from build123d import *

# Parameters (mm, degrees)
BOSS_EXTRUDE1_DEPTH = 92
BOSS_EXTRUDE2_DEPTH = 11
BOSS_EXTRUDE3_DEPTH = 5
CUT_EXTRUDE1_REACH  = 91.375
SKETCH4_R           = 1.05
BOSS_EXTRUDE4_DEPTH = 11
CUT_EXTRUDE2_DEPTH  = 6.153427125
CUT_EXTRUDE3_REACH  = 96.249
SKETCH7_R           = 1.05
CHAMFER2_SIZE       = 2


with BuildPart() as part:
    # Sketch1 → Boss-Extrude1 (new body)
    with BuildSketch(Plane(origin=(0, 0, 0), x_dir=(1, 0, 0), z_dir=(0, 1, 0))):
        Polygon((0, 15.628427125), (-2.5, 15.628427125), (-13.153427125, 4.975), (-13.153427125, -5.025), (-2.5, -15.678427125), (0, -15.678427125), (0, -7.725), (-7.675, -7.725), (-7.675, 7.625), (0, 7.625), align=None)
    extrude(amount=BOSS_EXTRUDE1_DEPTH)

    # Sketch2 → Boss-Extrude2 (add)
    with BuildSketch(Plane.XZ):
        with BuildLine():
            Line((0, 7.725), (0, 5.075))
            ThreePointArc((0, 5.075), (-5.075, 0), (0, -5.075))
            Line((0, -5.075), (0, -7.625))
            Line((0, -7.625), (-7.675, -7.625))
            Line((-7.675, -7.625), (-7.675, 7.725))
            Line((-7.675, 7.725), (0, 7.725))
        make_face()
    extrude(amount=-BOSS_EXTRUDE2_DEPTH)

    # Sketch3 → Boss-Extrude3 (add)
    with BuildSketch(Plane(origin=(0, 92, 0), x_dir=(1, 0, 0), z_dir=(0, 1, 0))):
        Polygon((-2.5, 15.628427125), (-13.153427125, 15.628427125), (-13.153427125, 4.975), align=None)
        Polygon((-2.5, -15.678427125), (-13.153427125, -15.678427125), (-13.153427125, -5.025), align=None)
    extrude(amount=-BOSS_EXTRUDE3_DEPTH)

    # Sketch4 → Cut-Extrude1 (cut, up to next)
    with BuildSketch(Plane.XZ.offset(-87), mode=Mode.PRIVATE) as cut_extrude1_sk1:
        with Locations(Location((-10.153427125, 12.678427125, 0), (0, 0, 270))):
            Circle(SKETCH4_R)
    cut_extrude1_tool1 = extrude(cut_extrude1_sk1.sketch, amount=-CUT_EXTRUDE1_REACH, mode=Mode.PRIVATE) & part.part
    # Sketch4 → Cut-Extrude1 (cut, up to next)
    with BuildSketch(Plane.XZ.offset(-87), mode=Mode.PRIVATE) as cut_extrude1_sk2:
        with Locations(Location((-10.153427125, -12.628427125, 0), (0, 0, 270))):
            Circle(SKETCH4_R)
    cut_extrude1_tool2 = extrude(cut_extrude1_sk2.sketch, amount=-CUT_EXTRUDE1_REACH, mode=Mode.PRIVATE) & part.part
    add(cut_extrude1_tool1.solids().sort_by_distance((-10.153427, 87, 12.678427))[0], mode=Mode.SUBTRACT)
    add(cut_extrude1_tool2.solids().sort_by_distance((-10.153427, 87, -12.628427))[0], mode=Mode.SUBTRACT)

    # Sketch5 → Boss-Extrude4 (add)
    with BuildSketch(Plane.XZ):
        Polygon((-2.5, 15.678427125), (-13.153427125, 15.678427125), (-13.153427125, 5.025), align=None)
        Polygon((-13.153427125, -4.975), (-13.153427125, -15.628427125), (-2.5, -15.628427125), align=None)
    extrude(amount=-BOSS_EXTRUDE4_DEPTH)

    # Sketch6 → Cut-Extrude2 (cut)
    with BuildSketch(Plane.ZY.offset(13.153427125)):
        Polygon((11.564149128, 7.6), (9.139277997, 7.6), (7.926842432, 5.5), (9.139277997, 3.4), (11.564149128, 3.4), (12.776584693, 5.5), align=None)
        Polygon((-7.876842432, 5.5), (-9.089277997, 7.6), (-11.514149128, 7.6), (-12.726584693, 5.5), (-11.514149128, 3.4), (-9.089277997, 3.4), align=None)
    extrude(amount=-CUT_EXTRUDE2_DEPTH, mode=Mode.SUBTRACT)

    # Sketch7 → Cut-Extrude3 (cut, up to next)
    with BuildSketch(Plane.ZY.offset(13.153427125), mode=Mode.PRIVATE) as cut_extrude3_sk1:
        with Locations((-10.301713562, 5.5)):
            Circle(SKETCH7_R)
    cut_extrude3_tool1 = extrude(cut_extrude3_sk1.sketch, amount=-CUT_EXTRUDE3_REACH, mode=Mode.PRIVATE) & part.part
    # Sketch7 → Cut-Extrude3 (cut, up to next)
    with BuildSketch(Plane.ZY.offset(13.153427125), mode=Mode.PRIVATE) as cut_extrude3_sk2:
        with Locations((10.351713562, 5.5)):
            Circle(SKETCH7_R)
    cut_extrude3_tool2 = extrude(cut_extrude3_sk2.sketch, amount=-CUT_EXTRUDE3_REACH, mode=Mode.PRIVATE) & part.part
    add(cut_extrude3_tool1.solids().sort_by_distance((-13.153427, 5.5, -10.301714))[0], mode=Mode.SUBTRACT)
    add(cut_extrude3_tool2.solids().sort_by_distance((-13.153427, 5.5, 10.351714))[0], mode=Mode.SUBTRACT)

    # Chamfer2
    # the kernel refuses this chamfer: 2 mm, written as the material it takes off along each edge
    with BuildSketch(Plane(origin=(-7, 5.5, 10.351713562), x_dir=(0, 0, 1), z_dir=(0, -1, 0))) as chamfer2_piece_1_section:
        Polygon((1.05, -CHAMFER2_SIZE), (1.05 + CHAMFER2_SIZE, 0), (1.05, 0), align=None)
    chamfer2_piece_1 = revolve(axis=Axis((-7, 5.5, 10.351713562), (-1, 0, 0)), mode=Mode.PRIVATE)
    chamfer2_piece_1 = split(chamfer2_piece_1, bisect_by=Plane(origin=(-5.677336613, 7.282209745, 11.747625417), z_dir=(2.5539348178531628e-15, -0.5000000000000006, -0.8660254037844384)), keep=Keep.TOP, mode=Mode.PRIVATE)
    chamfer2_piece_1 = split(chamfer2_piece_1, bisect_by=Plane(origin=(-5.677336613, 3.717790255, 11.747625417), z_dir=(2.553934817853164e-15, 0.5000000000000003, -0.8660254037844387)), keep=Keep.TOP, mode=Mode.PRIVATE)
    chamfer2_piece_1 = split(chamfer2_piece_1, bisect_by=Plane(origin=(-5.677336613, 3.4, 8.660747588), z_dir=(0, 1, 0)), keep=Keep.TOP, mode=Mode.PRIVATE)
    chamfer2_piece_1 = split(chamfer2_piece_1, bisect_by=Plane(origin=(-5.677336613, 5.182209745, 8.110318721), z_dir=(-2.5539348178531624e-15, 0.5000000000000008, 0.8660254037844383)), keep=Keep.TOP, mode=Mode.PRIVATE)
    chamfer2_piece_1 = split(chamfer2_piece_1, bisect_by=Plane(origin=(-5.677336613, 5.817790255, 8.110318721), z_dir=(-2.5539348178531624e-15, -0.5000000000000007, 0.8660254037844384)), keep=Keep.TOP, mode=Mode.PRIVATE)
    chamfer2_piece_1 = split(chamfer2_piece_1, bisect_by=Plane(origin=(-5.677336613, 7.6, 8.660747588), z_dir=(0, -1, 0)), keep=Keep.TOP, mode=Mode.PRIVATE)
    add(chamfer2_piece_1, mode=Mode.SUBTRACT)
    with BuildSketch(Plane(origin=(-7, 5.5, -10.301713562), x_dir=(0, 0, 1), z_dir=(0, -1, 0))) as chamfer2_piece_2_section:
        Polygon((1.05, -CHAMFER2_SIZE), (1.05 + CHAMFER2_SIZE, 0), (1.05, 0), align=None)
    chamfer2_piece_2 = revolve(axis=Axis((-7, 5.5, -10.301713562), (-1, 0, 0)), mode=Mode.PRIVATE)
    chamfer2_piece_2 = split(chamfer2_piece_2, bisect_by=Plane(origin=(-5.677336613, 3.717790255, -8.905801708), z_dir=(2.5539348178531635e-15, 0.5000000000000004, -0.8660254037844385)), keep=Keep.TOP, mode=Mode.PRIVATE)
    chamfer2_piece_2 = split(chamfer2_piece_2, bisect_by=Plane(origin=(-5.677336613, 3.4, -11.992679537), z_dir=(0, 1, 0)), keep=Keep.TOP, mode=Mode.PRIVATE)
    chamfer2_piece_2 = split(chamfer2_piece_2, bisect_by=Plane(origin=(-5.677336613, 5.182209745, -12.543108404), z_dir=(-2.5539348178531647e-15, 0.49999999999999933, 0.866025403784439)), keep=Keep.TOP, mode=Mode.PRIVATE)
    chamfer2_piece_2 = split(chamfer2_piece_2, bisect_by=Plane(origin=(-5.677336613, 5.817790255, -12.543108404), z_dir=(-2.5539348178531624e-15, -0.5000000000000007, 0.8660254037844384)), keep=Keep.TOP, mode=Mode.PRIVATE)
    chamfer2_piece_2 = split(chamfer2_piece_2, bisect_by=Plane(origin=(-5.677336613, 7.6, -11.992679537), z_dir=(0, -1, 0)), keep=Keep.TOP, mode=Mode.PRIVATE)
    chamfer2_piece_2 = split(chamfer2_piece_2, bisect_by=Plane(origin=(-5.677336613, 7.282209745, -8.905801708), z_dir=(2.553934817853164e-15, -0.5000000000000002, -0.8660254037844386)), keep=Keep.TOP, mode=Mode.PRIVATE)
    add(chamfer2_piece_2, mode=Mode.SUBTRACT)


solid = part.part
For this review, take the finished solid that the model builds, in its own axes (mm). A direction names the side the tool comes from. Round coordinates to 2 decimals unless told otherwise and drop trailing zeros. Loops run counter-clockwise (first coordinate to the right, second up) from the corner with the lowest first, then second, coordinate; pieces in that order, holes last. Notation, with made-up numbers: (-5.75, -21) - (-1.75, -21) arc R20 cw to (-1.75, 17) - close; hole circle Ø9 at (-38.75, 9.5). An arc over 180 degrees is marked (long way). One line per question, with ' | ' between items.
Q1. The part is to be moulded in two halves that separate along Y. For faces 4 (the flat face through (-8, 92, 0)), 5 (the flat face through (-9, 11, 12)), 6 (the cylindrical face through (-9.84, 89.46, -13.63)), 7 (the flat face through (-7, 0, 0)), say which applies: released by +Y, released by -Y, zero draft, split by the parting line, or undercut.
Taken from the geometry:
face 4: released by +Y | face 5: undercut | face 6: zero draft | face 7: released by -Y
Q2. Take a section at B-B (x = -1.5). Give the boundary of the cut face in (y, z) (3 decimals), and give its area (3 significant figures).
Taken from the geometry:
outline: (0, -15.628) - (92, -15.628) - (92, -7.625) - (11, -7.625) - (11, -4.848) - (0, -4.848) - close; (0, 4.848) - (11, 4.848) - (11, 7.725) - (92, 7.725) - (92, 15.678) - (0, 15.678) - close; hole circle Ø2.1 at (5.5, -10.302); hole circle Ø2.1 at (5.5, 10.352) | area: 1,520 mm²
Q3. Take a section at A-A (y = 78). Give the boundary of the cut face in (x, z) (3 decimals), and give its area (3 significant figures).
Taken from the geometry:
outline: (-13.153, -4.975) - (-2.5, -15.628) - (0, -15.628) - (0, -7.625) - (-7.675, -7.625) - (-7.675, 7.725) - (0, 7.725) - (0, 15.678) - (-2.5, 15.678) - (-13.153, 5.025) - close | area: 180 mm²
Q4. For line 1 along Z through (x, y) = (-9.75, 88); line 2 along Y through (x, z) = (-4.5, -6); line 3 along X through (y, z) = (47, 1.5) (3 decimals), list the stretches that pass through material, from the lowest coordinate up. Write a range as [from, to].
Taken from the geometry:
line 1: z = [-15.63, -13.6], [-11.66, 11.71], [13.65, 15.68] | line 2: y = [0, 11] | line 3: x = [-13.153, -7.675]
Q5. Take a section at C-C (z = 0). Give the boundary of the cut face in (x, y) (3 decimals).
Taken from the geometry:
outline: (-13.153, 0) - (-5.075, 0) - (-5.075, 11) - (-7.675, 11) - (-7.675, 92) - (-13.153, 92) - close
Q6. For pin 1 (5.5 mm diameter, centred on x = -8.5, z = -7.5, fed in from -Y); pin 2 (1 mm diameter, centred on x = -5.5, y = 24.5, fed in from -Z); pin 3 (1.9 mm diameter, centred on y = 5.5, z = 10.35, fed in from +X); pin 4 (2.5 mm diameter, centred on y = 5.5, z = -10.3, fed in from -X), all flat-tipped, find the tip position at first contact; note any pin that passes through.
Taken from the geometry:
pin 1: stops at y = 0 | pin 2: stops at z = -13.13 | pin 3: passes through | pin 4: stops at x = -5.2
Q7. Tool access review of faces 1 (the cylindrical face through (-9.838, 89.465, 11.677)), 2 (the flat face through (-10, 7.6, -10)), 3 (the flat face through (-7.9, 48.47, 10.28)): name each direction out of +Z, -Z, +X, -X, +Y, -Y from which nothing blocks a thin tool from reaching the whole face with its end or side.
Taken from the geometry:
face 1: +Y | face 2: -X | face 3: +Z, -X
